Design review of the part built by this model. Coordinates are the model's own, in mm. Face numbers are marked on the shaded views. Round coordinates to 2 decimals unless told otherwise and drop trailing zeros. Use CSV: the item, a comma, the result in double quotes. Start each with the question number.
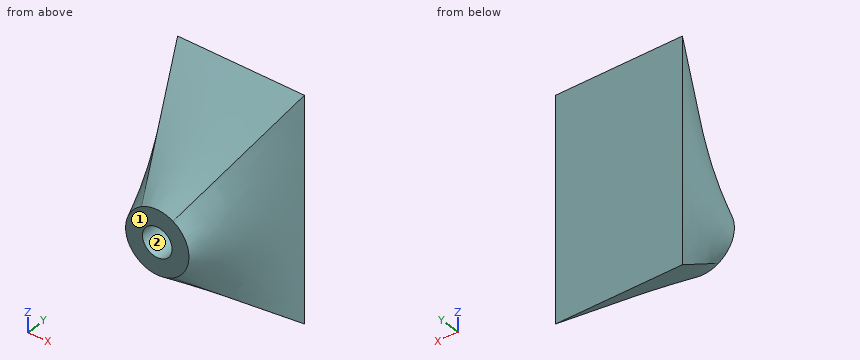
from build123d import *

# Parameters (mm, degrees)
SKETCH3_R          = 1.4
CUT_EXTRUDE1_DEPTH = 8


with BuildPart() as part:
    # Sketch1 for Loft2 → Loft2 section 0
    with BuildSketch(Plane(origin=(0, 0, 0), x_dir=(1, 0, 0), z_dir=(0, 1, 0))):
        with BuildLine():
            # circular arc as an exact rational Bezier (weights 1, cos(half-angle), 1)
            Bezier((-1.488416815, -2.604729426), (0, -3.455253321), (1.488416815, -2.604729426), weights=[1, 0.868243142, 1])
            Bezier((1.488416815, -2.604729426), (6.046693312, 0), (1.488416815, 2.604729426), weights=[1, 0.496138938, 1])
            Bezier((1.488416815, 2.604729426), (0, 3.455253321), (-1.488416815, 2.604729426), weights=[1, 0.868243142, 1])
            Bezier((-1.488416815, 2.604729426), (-6.046693312, 0), (-1.488416815, -2.604729426), weights=[1, 0.496138938, 1])
        make_face()
    # Sketch2 → Loft2 section 1
    with BuildSketch(Plane(origin=(0, 10, 0), x_dir=(1, 0, 0), z_dir=(0, 1, 0))):
        with BuildLine():
            Line((-6, -10.5), (6, -10.5))
            Line((6, -10.5), (6, 10.5))
            Line((6, 10.5), (-6, 10.5))
            Line((-6, 10.5), (-6, -10.5))
        make_face()
    loft()

    # Sketch3 → Cut-Extrude1 (cut)
    with BuildSketch(Plane(origin=(0, 0, 0), x_dir=(1, 0, 0), z_dir=(0, 1, 0))):
        with Locations(Location((0, 0, 0), (0, 0, 270))):
            Circle(SKETCH3_R)
    extrude(amount=CUT_EXTRUDE1_DEPTH, mode=Mode.SUBTRACT)


solid = part.part
Q1. Clearance check with flat-ended pins moving along their axes: pin 1 (5 mm diameter, centred on y = 4.5, z = -3.5, fed in from -X); pin 2 (2 mm diameter, centred on x = -2.5, y = 5, fed in from -Z); pin 3 (1 mm diameter, centred on x = -0.5, y = 2, fed in from +Z). State where each tip first meets the part, or that it passes through.
Q2. The part is to be moulded in two halves that separate along Z. For the marked faces 1 and 2, say which applies: +Z half, -Z half, draft (parallel to the pull), parting line (faces both ways), or undercut.
Q3. For L1, parallel to X at y = 5, z = 0; L2, parallel to X at y = 5.75, z = 0 (3 decimals); L3, parallel to Z at x = -0.5, y = 2.25, list the stretches that pass through material, from the lowest coordinate up. Write a range as [from, to].
Findings below:
1,pin 1,"stops at x = -5.01"
1,pin 2,"stops at z = -7.44"
1,pin 3,"stops at z = 4.86"
2,face 1,"draft"
2,face 2,"undercut"
3,L1,"x = [-4.5, -1.4], [1.4, 4.5]"
3,L2,"x = [-4.725, -1.4], [1.4, 4.725]"
3,L3,"z = [-4.68, -1.31], [1.31, 4.68]"
